```python
from build123d import *

# Parameters (mm, degrees)
SKETCH1_R           = 3
BOSS_EXTRUDE1_DEPTH = 4.7625
SKETCH2_R           = 14.2875
SKETCH2_R_2         = 3
BOSS_EXTRUDE2_DEPTH = 1.5875
SKETCH3_R           = 5
SKETCH3_R_2         = 3
BOSS_EXTRUDE3_DEPTH = 19.05
SKETCH4_R           = 4
CUT_EXTRUDE1_DEPTH  = 9.525


with BuildPart() as part:
    # Sketch1 → Boss-Extrude1 (new body)
    with BuildSketch(Plane.XY):
        with BuildLine():
            ThreePointArc((-3.568592622, 10.523915761), (0, 12.7), (3.568592622, 10.523915761))
            ThreePointArc((3.568592622, 10.523915761), (5.130117272, 8.885623765), (7.329682086, 8.352449747))
            ThreePointArc((7.329682086, 8.352449747), (10.998522628, 6.35), (10.898274707, 2.171466014))
            ThreePointArc((10.898274707, 2.171466014), (10.260234545, 0), (10.898274707, -2.171466014))
            ThreePointArc((10.898274707, -2.171466014), (10.998522628, -6.35), (7.329682086, -8.352449747))
            ThreePointArc((7.329682086, -8.352449747), (5.130117272, -8.885623765), (3.568592622, -10.523915761))
            ThreePointArc((3.568592622, -10.523915761), (0, -12.7), (-3.568592622, -10.523915761))
            ThreePointArc((-3.568592622, -10.523915761), (-5.130117272, -8.885623765), (-7.329682086, -8.352449747))
            ThreePointArc((-7.329682086, -8.352449747), (-10.998522628, -6.35), (-10.898274707, -2.171466014))
            ThreePointArc((-10.898274707, -2.171466014), (-10.260234545, 0), (-10.898274707, 2.171466014))
            ThreePointArc((-10.898274707, 2.171466014), (-10.998522628, 6.35), (-7.329682086, 8.352449747))
            ThreePointArc((-7.329682086, 8.352449747), (-5.130117272, 8.885623765), (-3.568592622, 10.523915761))
        make_face()
        Circle(SKETCH1_R, mode=Mode.SUBTRACT)
    extrude(amount=BOSS_EXTRUDE1_DEPTH)

    # Sketch2 → Boss-Extrude2 (add)
    with BuildSketch(Plane(origin=(0, 0, 0), x_dir=(-1, 0, 0), z_dir=(0, 0, -1))):
        Circle(SKETCH2_R)
        Circle(SKETCH2_R_2, mode=Mode.SUBTRACT)
    extrude(amount=BOSS_EXTRUDE2_DEPTH)

    # Sketch3 → Boss-Extrude3 (add)
    with BuildSketch(Plane.XY.offset(4.7625)):
        Circle(SKETCH3_R)
        Circle(SKETCH3_R_2, mode=Mode.SUBTRACT)
    extrude(amount=BOSS_EXTRUDE3_DEPTH)

    # Sketch4 → Cut-Extrude1 (cut)
    with BuildSketch(Plane.XY.offset(23.8125)):
        Circle(SKETCH4_R)
    extrude(amount=-CUT_EXTRUDE1_DEPTH, mode=Mode.SUBTRACT)


solid = part.part
```
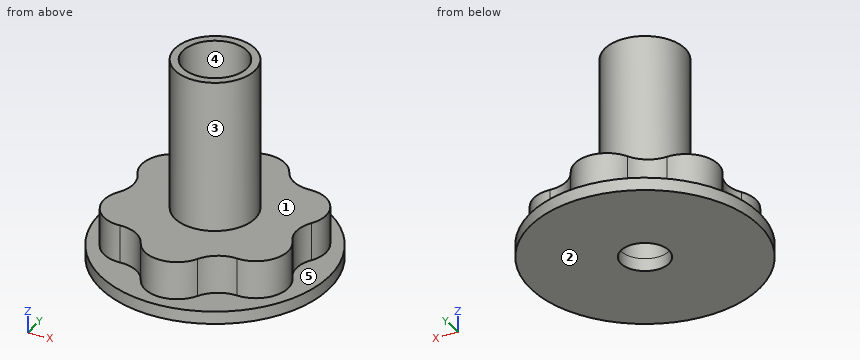
Can you work these out from the model? Positions are in its coordinate system, mm. Face numbers are marked on the shaded views. A direction names the side the tool comes from. Round coordinates to 2 decimals unless told otherwise and drop trailing zeros. Loops run counter-clockwise (first coordinate to the right, second up) from the corner with the lowest first, then second, coordinate; pieces in that order, holes last. Notation, with made-up numbers: M 78,57 L 87,57 A29 cw 87,86 Z; hole C 88.25,83 d9. An arc over 180 degrees is marked long. Answer as a JSON object with one key per item and string values. Group by question number.
Q1. Imagine slicing it at C-C, the plane z = 15.75. Please give me the cut outline in (x, y), then the cut area to 3 significant figures.
Q2. Will these pins go through, and if not, where does the flat tip stop? pin 1 (4 mm diameter, centred on x = -0.5, y = 1, fed in from +Z); pin 2 (8 mm diameter, centred on y = 0.5, z = 19, fed in from -X); pin 3 (4 mm diameter, centred on x = -6.5, y = -7, fed in from +Z).
Q3. On a 3-axis mill with a long thin cutter (end or side, diameter ignored), from which of +Z, -Z, +X, -X, +Y, -Y can I reach the whole of each face in a straight line? I mean the marked faces 1 and 2. Say none if no direction works.
Q4. Imagine slicing it at B-B, the plane x = 0. Please give me the cut outline in (y, z).
Q5. Please list where these lines run through material, in increasing order: L1, parallel to Y at x = 0, z = -0.4; L2, parallel to Y at x = 0, z = 9; L3, parallel to X at y = 0, z = 3.05.
Q6. We'd pull the mould along X, two halves only. Please class the marked faces 3, 4 and 5: +X half, -X half, draft (parallel to the pull), parting line (faces both ways), or undercut.
Q7. Imagine slicing it at A-A, the plane y = 0. Please give me the cut outline in (x, z).
Q8. Imagine slicing it at D-D, the plane z = 3.5. Please give me the cut outline in (x, y), then the cut area to 3 significant figures.
Findings:
{
 "1": {"outline": "C 0,0 d10; hole C 0,0 d8", "area": "28.3 mm2"},
 "2": {"pin 1": "stops at z = 14.29", "pin 2": "stops at x = -5", "pin 3": "stops at z = 4.76"},
 "3": {"face 1": "+Z", "face 2": "-Z, +X, -X, +Y, -Y"},
 "4": {"outline": "M -14.29,-1.59 L -3,-1.59 L -3,14.29 L -4,14.29 L -4,23.81 L -5,23.81 L -5,4.76 L -12.7,4.76 L -12.7,0 L -14.29,0 Z; M 3,-1.59 L 14.29,-1.59 L 14.29,0 L 12.7,0 L 12.7,4.76 L 5,4.76 L 5,23.81 L 4,23.81 L 4,14.29 L 3,14.29 Z"},
 "5": {"L1": "y = -14.29 to -3, 3 to 14.29", "L2": "y = -5 to -3, 3 to 5", "L3": "x = -10.26 to -3, 3 to 10.26"},
 "6": {"face 3": "parting line", "face 4": "undercut", "face 5": "draft"},
 "7": {"outline": "M -14.29,-1.59 L -3,-1.59 L -3,14.29 L -4,14.29 L -4,23.81 L -5,23.81 L -5,4.76 L -10.26,4.76 L -10.26,0 L -14.29,0 Z; M 3,-1.59 L 14.29,-1.59 L 14.29,0 L 10.26,0 L 10.26,4.76 L 5,4.76 L 5,23.81 L 4,23.81 L 4,14.29 L 3,14.29 Z"},
 "8": {"outline": "M -10.9,-2.17 A4.01 ccw -7.33,-8.35 A4.01 cw -3.57,-10.52 A4.01 ccw 3.57,-10.52 A4.01 cw 7.33,-8.35 A4.01 ccw 10.9,-2.17 A4.01 cw 10.9,2.17 A4.01 ccw 7.33,8.35 A4.01 cw 3.57,10.52 A4.01 ccw -3.57,10.52 A4.01 cw -7.33,8.35 A4.01 ccw -10.9,2.17 A4.01 cw Z; hole C 0,0 d6", "area": "394 mm2"}
}
